The listing builds one solid part. Answer for the finished solid, in the listing's coordinates (mm). Coordinates: 2 decimals unless noted, no trailing zeros. Order: outer loops, then holes, each group sorted by start corner. A loop starts at its lowest first (then second) coordinate and runs counter-clockwise, first axis right, second up. Notation, with made-up numbers: (-14.75, 7) - (-7.75, 7) arc R16 ccw to (-7.75, 27) - close; hole circle Ø10 at (73.25, 1.5). An arc over 180 degrees is marked (long way). One line per item, written item: value. Start each with the question number.
```python
from build123d import *

# Parameters (mm, degrees)
F1_DEPTH = 76.2
F2_R     = 11.632497
F3_DEPTH = 84.582


with BuildPart() as f1:
    # F0 (on Front) → F1 (new body)
    with BuildSketch(Plane.XZ):
        Polygon((41.046472, 38.463472), (-35.138952, 36.973097), (-33.648576, -39.212327), (42.536847, -37.721951), align=None)
    extrude(amount=F1_DEPTH)

    # F2 (on Front) → F3 (cut)
    with BuildSketch(Plane.XZ):
        Circle(F2_R)
    extrude(amount=F3_DEPTH, mode=Mode.SUBTRACT)


solid = f1.part
```
(1) Flat-ended cylindrical pins translate along their axes: pin 1 Ø6 at (y, z) = (-39.5, -3) entering from -X; pin 2 Ø5 at (y, z) = (-67.5, -21.5) entering from +X; pin 3 Ø8 at (y, z) = (-24, 21) entering from +X. Find the tip coordinate at first contact, or state that the pin passes through.
(2) Consider probe 1 along X at (y, z) = (-9, 5); probe 2 along Z at (x, y) = (8, -25); probe 3 along X at (y, z) = (-52, 0). Determine where each line is inside the solid, lowest interval first.
(3) The part is cut by section A-A on z = -7. Determine the outline of the cut face in (x, y).
(4) The part is cut by section D-D on x = 18.5. Determine the outline of the cut face in (y, z), plus the area to 3 significant figures.
(5) The part is cut by section C-C on y = -43.5. Determine the outline of the cut face in (x, z) (1 decimal), plus the area to 3 significant figures.
(6) The part is cut by section B-B on x = 0. Determine the outline of the cut face in (y, z).
(7) For a pull along Z with two mould halves and no side action, classify faces 1 (the face through (12, 0, 0)), 2 (the face through (11.095, -37.567, 3.494)) as pulls with the +Z half, pulls with the -Z half, needs draft (parallel to the pull), parting line crosses it, or undercut.
Completed:
1. pin 1: stops at x = -34.42
1. pin 2: stops at x = 42.27
1. pin 3: stops at x = 41.47
2. probe 1: x = -34.51 to -10.5, 10.5 to 41.7
2. probe 2: z = -38.4 to -8.44, 8.44 to 37.82
2. probe 3: x = -34.42 to -11.63, 11.63 to 41.8
3. outline: (-34.28, -76.2) - (-9.29, -76.2) - (-9.29, 0) - (-34.28, 0) - close; (9.29, -76.2) - (41.94, -76.2) - (41.94, 0) - (9.29, 0) - close
4. outline: (-76.2, -38.19) - (0, -38.19) - (0, 38.02) - (-76.2, 38.02) - close
4. area: 5,810 mm2
5. outline: (-35.1, 37) - (-33.6, -39.2) - (42.5, -37.7) - (41, 38.5) - close; hole circle Ø23.3 at (0, 0)
5. area: 5,380 mm2
6. outline: (-76.2, -38.55) - (0, -38.55) - (0, -11.63) - (-76.2, -11.63) - close; (-76.2, 11.63) - (0, 11.63) - (0, 37.66) - (-76.2, 37.66) - close
7. face 1: needs draft
7. face 2: undercut
